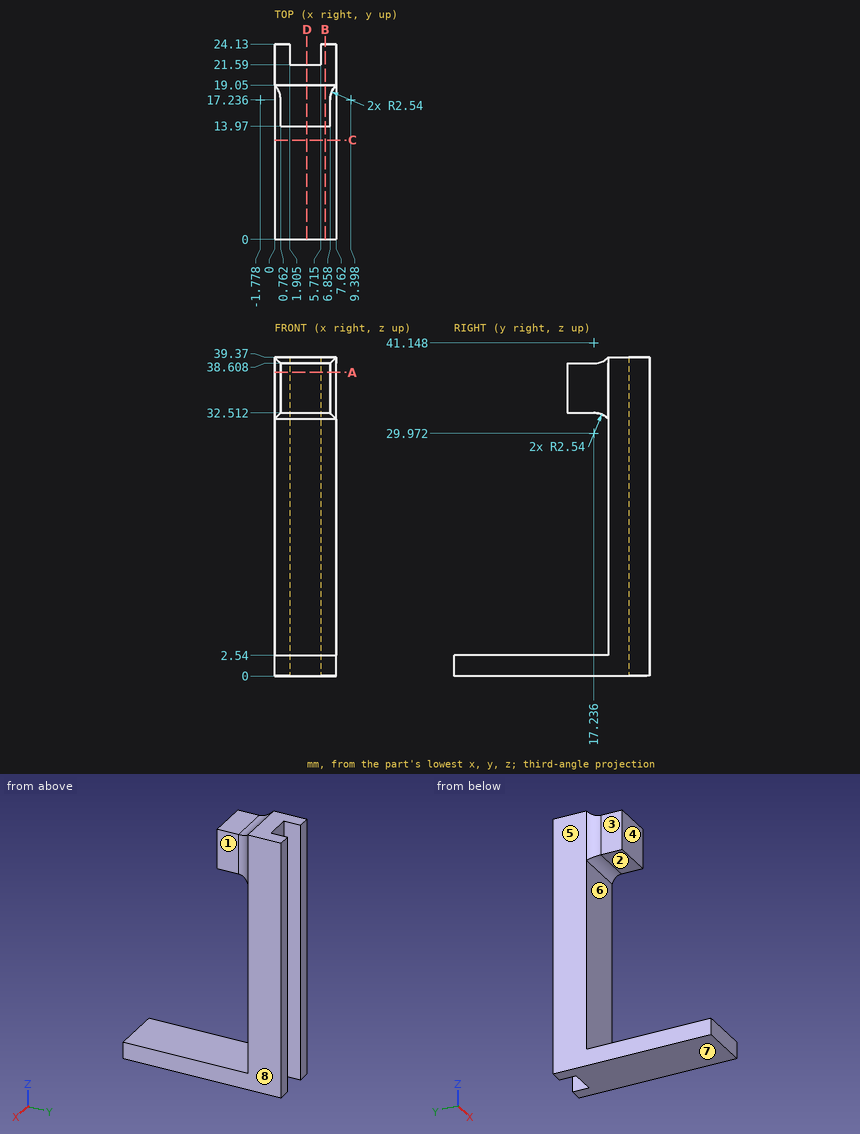
For this review, use the dimensioned drawing (mm, ordinates from the lowest corner) and the shaded views. A direction names the side the tool comes from. Round coordinates to 2 decimals unless told otherwise and drop trailing zeros. Order: outer loops, then holes, each group sorted by start corner. A loop starts at its lowest first (then second) coordinate and runs counter-clockwise, first axis right, second up. Notation, with made-up numbers: (41, 42.25) -> (52, 42.25) arc R20 ccw to (52, 78.25) -> close; hole circle Ø7 at (84.5, 0). An arc over 180 degrees is marked (long way). Use CSV: the item, a comma, the result in double quotes. Start each with the question number.
(1) Consider section B-B on x = 6.25. Write out the cut boundary in (y, z), and give its area (3 significant figures).
(2) Consider section C-C on y = 12.25. Write out the cut boundary in (x, z).
(3) Insertion check: pin 1 (1.8 mm diameter, centred on x = 4, z = 34, fed in from -Y); pin 2 (2.5 mm diameter, centred on x = 3.5, z = 15.5, fed in from -Y); pin 3 (4 mm diameter, centred on x = 1, y = 16, fed in from +Z). Each pin has a flat end and moves straight along its axis. Give the tip position at first contact, or say it passes through.
(4) Consider section D-D on x = 4. Write out the cut boundary in (y, z), and give its area (3 significant figures).
(5) Wall thickness on probe 1 along Z at (x, y) = (4, 15.5); probe 2 along X at (y, z) = (22.75, 11) (3 decimals); probe 3 along Y at (x, z) = (1.25, 33): over which ranges is each line inside the solid? List them lowest first. Write a range as from..to.
(6) Consider section A-A on z = 37.5. Write out the cut boundary in (x, y) (3 decimals).
(7) Mouldability with a two-part tool opening along Z and no side actions: class the marked faces 6, 7 and 8 as pulls with the +Z half, pulls with the -Z half, needs draft (parallel to the pull), parting line crosses it, or undercut.
(8) Tool access review of the marked faces 1, 2, 3, 4 and 5: name each direction out of +Z, -Z, +X, -X, +Y, -Y from which nothing blocks a thin tool from reaching the whole face with its end or side.
Responses:
1,outline,"(0, 0) -> (24.13, 0) -> (24.13, 39.37) -> (19.05, 39.37) arc R2.54 cw to (17.24, 38.61) -> (13.97, 38.61) -> (13.97, 32.51) -> (17.24, 32.51) arc R2.54 cw to (19.05, 31.75) -> (19.05, 2.54) -> (0, 2.54) -> close"
1,area,"280 mm²"
2,outline,"(0, 0) -> (7.62, 0) -> (7.62, 2.54) -> (0, 2.54) -> close"
3,pin 1,"y = 13.97"
3,pin 2,"y = 19.05"
3,pin 3,"z = 38.73"
4,outline,"(0, 0) -> (21.59, 0) -> (21.59, 39.37) -> (19.05, 39.37) arc R2.54 cw to (17.24, 38.61) -> (13.97, 38.61) -> (13.97, 32.51) -> (17.24, 32.51) arc R2.54 cw to (19.05, 31.75) -> (19.05, 2.54) -> (0, 2.54) -> close"
4,area,"180 mm²"
5,probe 1,"0..2.54, 32.51..38.61"
5,probe 2,"0..1.905, 5.715..7.62"
5,probe 3,"13.97..24.13"
6,outline,"(0, 19.05) arc R2.54 cw to (0.762, 17.236) -> (0.762, 13.97) -> (6.858, 13.97) -> (6.858, 17.236) arc R2.54 cw to (7.62, 19.05) -> (7.62, 24.13) -> (5.715, 24.13) -> (5.715, 21.59) -> (1.905, 21.59) -> (1.905, 24.13) -> (0, 24.13) -> close"
7,face 6,"undercut"
7,face 7,"pulls with the -Z half"
7,face 8,"needs draft"
8,face 1,"+Z, +X, -Y"
8,face 2,"+X, -X, -Y"
8,face 3,"+Z, -X, -Y"
8,face 4,"+Z, +X, -X, -Y"
8,face 5,"+Z, -Z, -X, +Y, -Y"
